from build123d import *

# Parameters (mm, degrees)
F0_R     = 13.5257644579
F1_DEPTH = 25
F2_SIZE  = 10
F3_DEPTH = 25
F4_R     = 1.3988438113
F5_DEPTH = 100


# Not quite as in the source:
# - a fillet or chamfer that OpenCascade refuses, or shapes differently, is made with other operations: its cross-section is extruded or revolved along the edge and cut away or added


with BuildPart() as f1:
    # F0 (on Top) → F1 (new body)
    with BuildSketch(Plane.XY):
        Circle(F0_R)
    extrude(amount=F1_DEPTH)

    # F2
    f2_edges = [f1.edges().sort_by_distance(p)[0] for p in [
        (-13.525764, 0, 25),
    ]]
    chamfer(f2_edges, length=F2_SIZE)

    # F3 (add): a face of the model
    f3_faces = [f1.faces().sort_by_distance(p)[0] for p in [
        (0, 0, 25),
    ]]
    extrude(f3_faces, amount=F3_DEPTH)

    # F4 (on face) → F5 (cut)
    with BuildSketch(Plane.XY.offset(50)):
        Circle(F4_R)
    extrude(amount=-F5_DEPTH, mode=Mode.SUBTRACT)

    # F6: chamfer of 3 on 1 edges, made by hand

    # F6_s1 → F6_t2 (revolve, cut)
    with BuildSketch(Plane.XZ):
        Polygon((3.5257644579, 47), (0.5257644579, 50), (3.5257644579, 50), align=None)
    revolve(axis=Axis((0, 0, 50), (0, 0, 1)), mode=Mode.SUBTRACT)


solid = f1.part
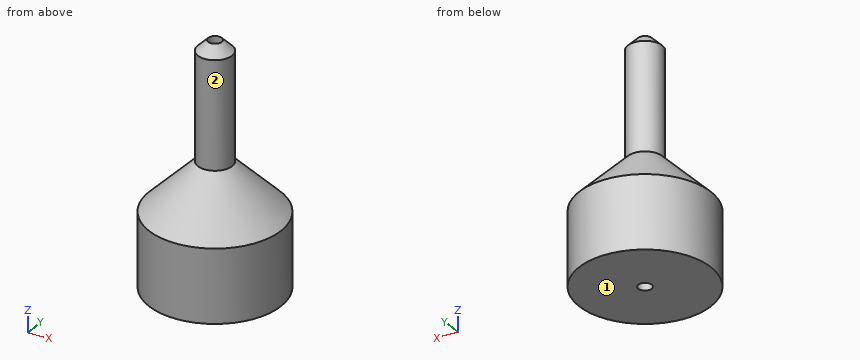
Part model, mm, in its own coordinate system. Face numbers are marked on the shaded views. A direction names the side the tool comes from. Round coordinates to 2 decimals unless told otherwise and drop trailing zeros. Loops run counter-clockwise (first coordinate to the right, second up) from the corner with the lowest first, then second, coordinate; pieces in that order, holes last. Notation, with made-up numbers: (-28.5, 24.25) - (13.5, 24.25) arc R27 ccw to (13.5, 48.25) - close; hole circle Ø10 at (-37.5, 53.5). An arc over 180 degrees is marked (long way). Answer as a JSON object with one key per item and string values.
Item 1: Pin check, flat tips, straight feed: pin 1 (2 mm diameter, centred on x = -5.5, y = 6.5, fed in from +Z); pin 2 (5 mm diameter, centred on x = 5.5, z = 25, fed in from +Y); pin 3 (5 mm diameter, centred on x = -7.5, y = -1.5, fed in from +Z). Stop position of each tip, or through.
Output:
{"pin 1": "z = 21.01", "pin 2": "y = 3.81", "pin 3": "z = 23.38"}
Item 2: Tool access for the marked faces 1 and 2: list every direction of +Z, -Z, +X, -X, +Y, -Y with a clear straight run to the whole face (end or side of a thin tool).
Output:
{"face 1": "-Z, +X, -X, +Y, -Y", "face 2": "+Z"}
Item 3: Band-saw the part on A-A on x = 0. List the corners of the cut face in (y, z).
Output:
{"outline": "(-13.53, 0) - (-1.4, 0) - (-1.4, 49.13) - (-3.53, 47) - (-3.53, 25) - (-13.53, 15) - close; (1.4, 0) - (13.53, 0) - (13.53, 15) - (3.53, 25) - (3.53, 47) - (1.4, 49.13) - close"}
Item 4: Wall check: L1, parallel to Y at x = 0, z = 35; L2, parallel to Y at x = 0, z = 19; L3, parallel to Z at x = -10.5, y = -4.5. Give the ranges that are in metal, low to high.
Output:
{"L1": "-3.53 to -1.4, 1.4 to 3.53", "L2": "-9.53 to -1.4, 1.4 to 9.53", "L3": "0 to 17.1"}
Item 5: Band-saw the part on C-C on z = 34. List the corners of the cut face in (x, y), plus the area to 3 significant figures.
Output:
{"outline": "circle Ø7.05 at (0, 0); hole circle Ø2.8 at (0, 0)", "area": "32.9 mm2"}
